For this review, take the finished solid that the model builds, in its own axes (mm). Give positions to 0.01 mm unless a question says otherwise; leave off trailing zeros. Write each loop counter-clockwise with the first axis right and the second up, starting at its lowest first coordinate (ties: lowest second). Pieces come first, ordered by that corner, then holes. Notation, with made-up numbers: M 77.5,-1.75 L 92.5,-1.75 A26 cw 92.5,21.25 Z; hole C 24,-12 d5. An arc over 180 degrees is marked long. Use one line per item in the form item = value. Start each with the question number.
Q1. Clearance check with flat-ended pins moving along their axes: pin 1 Ø1 at (x, z) = (678.5, 1) entering from -Y; pin 2 Ø0.6 at (y, z) = (1220.5, 1.5) entering from +X; pin 3 Ø5 at (x, y) = (548, 72.5) entering from -Z; pin 4 Ø0.6 at (y, z) = (1122.5, 1.5) entering from +X. State where each tip first meets the part, or that it passes through.
Q2. For probe 1 along X at (y, z) = (1024.5, 0.9), list the stretches that pass through material, from the lowest coordinate up. Write a range as [from, to].
Q3. Consider section A-A on y = 1109. Write out the cut boundary in (x, z).
Autodesk Inventor part; units mm, degrees
ref_plane "YZ Plane" through (0, 0, 0) normal (1, 0, 0) x (0, 1, 0)
ref_plane "XZ Plane" through (0, 0, 0) normal (0, 1, 0) x (-1, 0, 0)
ref_plane "XY Plane" through (0, 0, 0) normal (0, 0, 1) x (1, 0, 0)
sketch "Sketch1" plane through (0, 0, 0) normal (0, 0, 1) x (1, 0, 0)
  line L0 (-692.5, -1287.5) -> (692.5, -1287.5)
  line L1 (692.5, -1287.5) -> (692.5, 1287.5)
  line L2 (692.5, 1287.5) -> (-692.5, 1287.5)
  line L3 (-692.5, 1287.5) -> (-692.5, -1287.5)
  line L4 (-692.5, -1287.5) -> (692.5, 1287.5) construction
  line L5 (692.5, -1287.5) -> (-692.5, 1287.5) construction
  line L6 (692.5, -1247.5) -> (652.5, -1247.5)
  line L7 (652.5, -1247.5) -> (652.5, -1287.5)
  line L8 (692.5, 1222.5) -> (652.5, 1222.5)
  line L9 (652.5, 1222.5) -> (652.5, 932.5)
  line L10 (652.5, 932.5) -> (692.5, 932.5)
  line L11 (692.5, 932.5) -> (692.5, 1222.5)
  line L12 (652.5, 1067.5) -> (642.5, 1067.5)
  line L13 (642.5, 1067.5) -> (642.5, 1217.5)
  line L14 (642.5, 1217.5) -> (652.5, 1217.5)
  line L15 (-572.5, -767.5) -> (17.5, -767.5)
  line L16 (17.5, -767.5) -> (17.5, -177.5)
  line L17 (17.5, -177.5) -> (-572.5, -177.5)
  line L18 (-572.5, -177.5) -> (-572.5, -767.5)
  point P0 (0, 0)
  dimension "d154" = 1385
  dimension "d155" = 2575
  dimension "d157" = 40
  dimension "d159" = 290
  dimension "d161" = 40
  dimension "d162" = 2220
  dimension "d163" = 10
  dimension "d164" = 150
  dimension "d165" = 5
  dimension "d166" = 590
  dimension "d167" = 590
  dimension "d168" = 675
  dimension "d169" = 520
extrude "Plate5" add sketch "Sketch1" along normal blind 2 contours L3 L2 L1 L8 L9 L14 L13 L12 L10 L6 L7 L0 | L18 L17 L16 L15
fillet "Corner Round1" radius 15 1 edges at (652.5, -1247.5, 1)
properties part number "PNS-0111 floor sheet 2_CPY" material "Stainless Steel"
Working result:
q1.pin_1 = -1247.5
q1.pin_2 = 652.5
q1.pin_3 = 0
q1.pin_4 = 642.5
q2.probe_1 = [-692.5, 652.5]
q3.outline = M -692.5,0 L 642.5,0 L 642.5,2 L -692.5,2 Z
